from build123d import *

# Parameters (mm, degrees)
F1_DEPTH = 20
F2_R     = 5
F3_DEPTH = 2.001
F4_R     = 5
F5_DEPTH = 2.000768
F6_W     = 4
F6_H     = 5
F7_DEPTH = 2.000768
F8_R     = 1


with BuildPart() as f1:
    # F0 (on Front) → F1 (new body)
    with BuildSketch(Plane.XZ):
        with BuildLine():
            Line((0, 2), (0, 0))
            Line((0, 0), (29, 0))
            ThreePointArc((29, 0), (29.707107, 0.292893), (30, 1))
            Line((30, 1), (30, 30))
            Line((30, 30), (28.000232, 29.969506))
            Line((28.000232, 29.969506), (28.000232, 3))
            ThreePointArc((28.000232, 3), (27.707339, 2.292893), (27.000232, 2))
            Line((27.000232, 2), (0, 2))
        make_face()
    extrude(amount=-F1_DEPTH)

    # F2 (on face) → F3 (cut, through all)
    with BuildSketch(Plane.XY.offset(2)):
        with Locations((10, 10)):
            Circle(F2_R)
    extrude(amount=-F3_DEPTH, mode=Mode.SUBTRACT)

    # F4 (on face) → F5 (cut, through all)
    with BuildSketch(Plane(origin=(28.000232, 0, 0), x_dir=(0, -1, 0), z_dir=(-1, 0, 0))):
        with Locations((-10, 19.969506)):
            Circle(F4_R)
    extrude(amount=-F5_DEPTH, mode=Mode.SUBTRACT)

    # F6 (on face) → F7 (cut, through all)
    with BuildSketch(Plane(origin=(28.000232, 0, 0), x_dir=(0, -1, 0), z_dir=(-1, 0, 0))):
        with Locations((-2, 7.469506)):
            Rectangle(F6_W, F6_H)
    extrude(amount=-F7_DEPTH, mode=Mode.SUBTRACT)

    # F8
    f8_edges = [f1.edges().sort_by_distance(p)[0] for p in [
        (0, 0, 1),
        (29.000116, 0, 29.984753),
        (0, 20, 1),
        (29.000116, 20, 29.984753),
    ]]
    fillet(f8_edges, radius=F8_R)


solid = f1.part
Read the model definition and answer for the solid it produces. Units are mm, in the model's axes. A direction names the side the tool comes from. Coordinates: 2 decimals unless noted, no trailing zeros. Loops run counter-clockwise (first coordinate to the right, second up) from the corner with the lowest first, then second, coordinate; pieces in that order, holes last. Notation, with made-up numbers: (35.25, -10.5) -> (74.25, -10.5) arc R9 ccw to (74.25, -0.5) -> close; hole circle Ø8 at (57, -8.5). An arc over 180 degrees is marked (long way). Write item = value, one per line. Start each with the question number.
1) The part is cut by section A-A, the plane x = 10. Determine the outline of the cut face in (y, z).
2) The mould has two halves that part along Z. Classify faces 1 (the face through (29, 19.7, 29.7)), 2 (the face through (0, 10, 1)), 3 (the face through (28.986, 5.381, 18.054)): pulls with the +Z half, pulls with the -Z half, needs draft (parallel to the pull), parting line crosses it, or undercut.
3) The part is cut by section C-C, the plane y = 7.75. Determine the outline of the cut face in (x, z).
4) For faces 4 (the face through (28, 10, 14)), 5 (the face through (0.285, 19.699, 0.986)), 6 (the face through (29, 4, 7)), determine the directions among +Z, -Z, +X, -X, +Y, -Y from which every point of the face is accessible in a straight line to the end or side of a thin tool.
5) Given P1, Ø6, axis at y = 10, z = 23, coming from the -X side; P2, Ø5, axis at x = 5.5, y = 2.5, coming from the +Z side; P3, Ø2, axis at x = 29, z = 7.5, coming from the -Y side, each flat-ended and moving along its own axis, determine where each tip first touches the part or whether it passes through.
6) The part is cut by section B-B, the plane y = 1.5. Determine the outline of the cut face in (x, z), plus the area to 3 significant figures.
7) Find the intervals of material crossed by L1, parallel to Y at x = 10, z = 1; L2, parallel to X at y = 16, z = 23; L3, parallel to Z at x = 13, y = 3.25, in increasing order. Write a range as from..to.
8) The part is cut by section D-D, the plane z = 21. Determine the outline of the cut face in (x, y).
Result:
q1.outline = (0, 0) -> (5, 0) -> (5, 2) -> (0, 2) -> close; (15, 0) -> (20, 0) -> (20, 2) -> (15, 2) -> close
q2.face_1 = pulls with the +Z half
q2.face_2 = needs draft
q2.face_3 = undercut
q3.outline = (0, 0) -> (5.53, 0) -> (5.53, 2) -> (0, 2) -> close; (14.47, 0) -> (29, 0) arc R1 ccw to (30, 1) -> (30, 15.5) -> (28, 15.5) -> (28, 3) arc R1 cw to (27, 2) -> (14.47, 2) -> close; (28, 24.43) -> (30, 24.43) -> (30, 30) -> (28, 29.97) -> close
q4.face_4 = +Z, -X, +Y, -Y
q4.face_5 = +Z, -Z, -X, +Y
q4.face_6 = +X, -X, -Y
q5.P1 = 28
q5.P2 = 2
q5.P3 = 4
q6.outline = (0, 0) -> (29, 0) arc R1 ccw to (30, 1) -> (30, 4.97) -> (28, 4.97) -> (28, 3) arc R1 cw to (27, 2) -> (0, 2) -> close; (28, 9.97) -> (30, 9.97) -> (30, 30) -> (28, 29.97) -> close
q6.area = 106 mm²
q7.L1 = 0..5, 15..20
q7.L2 = 28..30
q7.L3 = 0..2
q8.outline = (28, 0) -> (30, 0) -> (30, 5.11) -> (28, 5.11) -> close; (28, 14.89) -> (30, 14.89) -> (30, 20) -> (28, 20) -> close
